Here's how the part is built. I have some questions about the finished solid (model axes, mm). Give positions to 0.01 mm unless a question says otherwise; leave off trailing zeros. Order: outer loops, then holes, each group sorted by start corner. A loop starts at its lowest first (then second) coordinate and runs counter-clockwise, first axis right, second up.
from build123d import *

# Parameters (mm, degrees)
SKETCH1_W           = 15
SKETCH1_H           = 8
BOSS_EXTRUDE1_DEPTH = 5
SKETCH2_W           = 15
SKETCH2_H           = 2.5
BOSS_EXTRUDE2_DEPTH = 10
SKETCH4_R           = 1
CUT_EXTRUDE1_DEPTH  = 22.118712082
FILLET1_R           = 2.5


with BuildPart() as part:
    # Sketch1 → Boss-Extrude1 (new body)
    with BuildSketch(Plane.XY):
        Rectangle(SKETCH1_W, SKETCH1_H)
    extrude(amount=BOSS_EXTRUDE1_DEPTH)

    # Sketch2 → Boss-Extrude2 (add)
    with BuildSketch(Plane.XZ.offset(4)):
        with Locations((0, 3.75)):
            Rectangle(SKETCH2_W, SKETCH2_H)
    extrude(amount=BOSS_EXTRUDE2_DEPTH)

    # Sketch4 → Cut-Extrude1 (cut, through all)
    with BuildSketch(Plane(origin=(7.5, 0, 0), x_dir=(0, 0, -1), z_dir=(1, 0, 0))):
        with Locations((-2.5, 1.5)):
            Circle(SKETCH4_R)
    extrude(amount=-CUT_EXTRUDE1_DEPTH, mode=Mode.SUBTRACT)

    # Fillet1
    fillet1_edges = [part.edges().sort_by_distance(p)[0] for p in [
        (0, -14, 5),
        (0, 4, 0),
        (0, 4, 5),
    ]]
    fillet(fillet1_edges, radius=FILLET1_R - 0.0001)  # a hair under: the kernel refuses the full size


solid = part.part
Q1. If we section it at C-C on y = 2: List the corners of the cut face in (x, z) for me.
Filled sheet:
outline: (-7.5, 0.05) - (7.5, 0.05) - (7.5, 1.63) - (-7.5, 1.63) - close; (-7.5, 3.37) - (7.5, 3.37) - (7.5, 4.95) - (-7.5, 4.95) - close
Q2. Thinking about a two-plate mould opening in Z: for faces 1 (the face through (0, -4, 1)), 2 (the face through (0, -9, 2.5)), 3 (the face through (0.1, 0.9, 3.3)), 4 (the face through (0.105, -13.287, 4.248)), which applies, released by +Z, released by -Z, zero draft, split by the parting line, or undercut?
Filled sheet:
face 1: zero draft
face 2: released by -Z
face 3: undercut
face 4: released by +Z
Q3. If we section it at B-B on z = 1.9: List the corners of the cut face in (x, y) for me.
Filled sheet:
outline: (-7.5, -4) - (7.5, -4) - (7.5, 0.7) - (-7.5, 0.7) - close; (-7.5, 2.3) - (7.5, 2.3) - (7.5, 3.93) - (-7.5, 3.93) - close
Q4. I'm going to push a flat-ended pin straight in: P1, Ø3, axis at x = -3, y = -9, coming from the -Z side. Where does the tip first touch, or does it pass through?
Filled sheet:
P1: stops at z = 2.5
Q5. If we section it at D-D on y = -6.5: List the corners of the cut face in (x, z) for me.
Filled sheet:
outline: (-7.5, 2.5) - (7.5, 2.5) - (7.5, 5) - (-7.5, 5) - close
Q6. I need wall thicknesses on L1, parallel to Y at x = -0.25, z = 3.1; L2, parallel to Y at x = -2.5, z = 3.2; L3, parallel to Z at x = 1.5, y = -6.75. Which ranges of each line are inside material? Lowest first, please.
Filled sheet:
L1: y = -13.93 to 0.7, 2.3 to 3.93
L2: y = -13.9 to 0.79, 2.21 to 3.9
L3: z = 2.5 to 5
